Autodesk Inventor part; units mm, degrees
ref_plane "YZ Plane" through (0, 0, 0) normal (1, 0, 0) x (0, 1, 0)
ref_plane "XZ Plane" through (0, 0, 0) normal (0, 1, 0) x (-1, 0, 0)
ref_plane "XY Plane" through (0, 0, 0) normal (0, 0, 1) x (1, 0, 0)
sketch "Sketch1" plane through (0, 0, 0) normal (0, 0, 1) x (1, 0, 0)
  line L0 (0, -7.3323) -> (-6.35, -3.6662)
  line L1 (-6.35, -3.6662) -> (-6.35, 3.6662)
  line L2 (-6.35, 3.6662) -> (0, 7.3323)
  line L3 (0, 7.3323) -> (6.35, 3.6662)
  line L4 (6.35, 3.6662) -> (6.35, -3.6662)
  line L5 (6.35, -3.6662) -> (0, -7.3323)
  circle A0 centre (0, 0) radius 3
  dimension "d0" = 12.7
  dimension "d1" = 6
extrude "Extrusion2" add sketch "Sketch1" along normal mid plane 58.5 contours L0 L1 L2 L3 L4 L5 | A0
sketch "Sketch4" plane through (-6.35, -3.6662, -29.25) normal (-1, 0, 0) x (0, 0, 1)
  line L0 (58.5, 7.3323) -> (58.5, 0)
  line L1 (0, 0) -> (0, 7.3323)
  point P0 (29.25, 3.6662)
  point P1 (29.25, 3.6662)
  point P2 (58.5, 3.6662)
  dimension "d43" = 58.5
hole "Hole4" at (-6.35, 0, 0) direction (1, 0, 0) diameter 6 end through all
sketch "Sketch5" plane through (0, 0, -29.25) normal (0, 0, -1) x (-1, 0, 0)
  point P0 (0, 0)
  point P1 (0, 0)
hole "Hole5" at (0, 0, -29.25) direction (0, 0, 1) diameter 4.917 depth 17.1 tip angle 118
mirror "Mirror1" about plane through (0, 0, 0) normal (0, 0, 1) of "Hole5"
properties part number "pistony"
Could you check a few things on this model? Use its own coordinates, in mm. A direction names the side the tool comes from. Give positions to 0.01 mm unless a question says otherwise; leave off trailing zeros. Order: outer loops, then holes, each group sorted by start corner. A loop starts at its lowest first (then second) coordinate and runs counter-clockwise, first axis right, second up.
Item 1: If we section it at D-D, the plane z = -6.5: Write out the boundary of the cut face in (x, y), plus the area to 3 significant figures.
Item 2: If we section it at A-A, the plane z = 0: Write out the boundary of the cut face in (x, y).
Item 3: If we section it at B-B, the plane z = 18: Write out the boundary of the cut face in (x, y), plus the area to 3 significant figures.
Item 4: I'm going to push flat-ended pins straight in: pin 1 (6 mm diameter, centred on y = 4, z = -4, fed in from +X); pin 2 (4.5 mm diameter, centred on x = 0, y = 0, fed in from -Z); pin 3 (1.5 mm diameter, centred on y = -5, z = -10, fed in from +X); pin 4 (4 mm diameter, centred on x = -4.5, z = 7, fed in from -Y). Where does each tip first touch, or does it pass through?
Item 5: If we mould it in two halves opening along X, with no side actions, what happens to faces 1 (the face through (0.13, 0.41, -10.93)), 2 (the face through (0, 0, -3)), 3 (the face through (-3.219, 5.474, 0.41))? For each: pulls with the +X half, pulls with the -X half, needs draft (parallel to the pull), parting line crosses it, or undercut.
Item 6: If we section it at C-C, the plane x = -3.75: Write out the boundary of the cut face in (y, z), plus the area to 3 significant figures.
Item 7: I need wall thicknesses on line 1 (X direction, y = 0, z = 17.5). Which ranges of the line are inside material? Lowest first, please.
Item 8: For faces 4 (the face through (0.738, 2.345, 20.58)), 5 (the face through (6.35, -3.2, 0.4)), 6 (the face through (-0.738, 2.345, -20.58)), which set-ups out of +Z, -Z, +X, -X, +Y, -Y let a thin tool reach every point of the face, with its end or its side?
Values:
1. outline: (-6.35, -3.67) - (0, -7.33) - (6.35, -3.67) - (6.35, 3.67) - (0, 7.33) - (-6.35, 3.67) - close
1. area: 140 mm2
2. outline: (-6.35, -3.67) - (0, -7.33) - (6.35, -3.67) - (6.35, -3) - (-6.35, -3) - close; (-6.35, 3) - (6.35, 3) - (6.35, 3.67) - (0, 7.33) - (-6.35, 3.67) - close
3. outline: (-6.35, -3.67) - (0, -7.33) - (6.35, -3.67) - (6.35, 3.67) - (0, 7.33) - (-6.35, 3.67) - close; hole circle Ø4.92 at (0, 0)
3. area: 121 mm2
4. pin 1: stops at x = 6.35
4. pin 2: stops at z = -12.02
4. pin 3: stops at x = 5.34
4. pin 4: stops at y = -5.89
5. face 1: undercut
5. face 2: needs draft
5. face 3: pulls with the -X half
6. outline: (-5.17, -29.25) - (5.17, -29.25) - (5.17, 29.25) - (-5.17, 29.25) - close; hole circle Ø6 at (0, 0)
6. area: 576 mm2
7. line 1: x = -6.35 to -2.46, 2.46 to 6.35
8. face 4: +Z
8. face 5: +Z, -Z, +X, +Y, -Y
8. face 6: -Z
